For this review, take the finished solid that the model builds, in its own axes (mm). Face numbers are marked on the shaded views. A direction names the side the tool comes from. Give positions to 0.01 mm unless a question says otherwise; leave off trailing zeros. Loops run counter-clockwise (first coordinate to the right, second up) from the corner with the lowest first, then second, coordinate; pieces in that order, holes last.
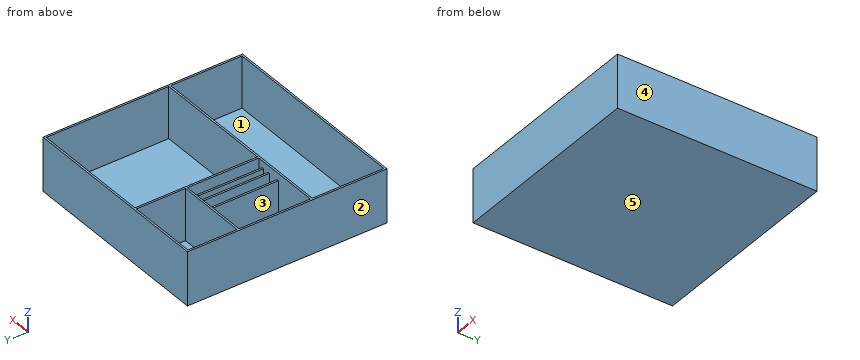
```python
from build123d import *

# Parameters (mm, degrees)
F0_W     = 92
F0_H     = 63.4
F1_DEPTH = 2.4
F0_W_2   = 56.8
F0_H_2   = 92
F0_W_3   = 14
F0_W_4   = 8
F0_W_5   = 6
F0_W_6   = 252.2
F0_W_7   = 257
F0_H_3   = 257
F2_DEPTH = 69
F0_W_8   = 2.4
F3_DEPTH = 60


with BuildPart() as f1:
    # F0 (on Top) → F1 (new body)
    with BuildSketch(Plane.XY):
        with Locations((-80.1, 94.4)):
            Rectangle(F0_W, F0_H)
    extrude(amount=F1_DEPTH)



with BuildPart() as f1b:
    # F0 (on Top) → F1, piece 2 (new body)
    with BuildSketch(Plane.XY):
        with Locations((-97.7, 14.3)):
            Rectangle(F0_W_2, F0_H_2)
    extrude(amount=F1_DEPTH)


with BuildPart() as f1c:
    # F0 (on Top) → F1, piece 3 (new body)
    with BuildSketch(Plane.XY):
        with Locations((-59.9, 14.3)):
            Rectangle(F0_W_3, F0_H_2)
    extrude(amount=F1_DEPTH)


with BuildPart() as f1d:
    # F0 (on Top) → F1, piece 4 (new body)
    with BuildSketch(Plane.XY):
        with Locations((-46.5, 14.3)):
            Rectangle(F0_W_4, F0_H_2)
    extrude(amount=F1_DEPTH)


with BuildPart() as f1e:
    # F0 (on Top) → F1, piece 5 (new body)
    with BuildSketch(Plane.XY):
        with Locations((-37.1, 14.3)):
            Rectangle(F0_W_5, F0_H_2)
    extrude(amount=F1_DEPTH)


with BuildPart() as f1f:
    # F0 (on Top) → F1, piece 6 (new body)
    with BuildSketch(Plane.XY):
        Polygon((126.1, 126.1), (-31.7, 126.1), (-31.7, 60.3), (-31.7, -31.7), (126.1, -31.7), align=None)
    extrude(amount=F1_DEPTH)


with BuildPart() as f1g:
    # F0 (on Top) → F1, piece 7 (new body)
    with BuildSketch(Plane.XY):
        with Locations((0, -80.1)):
            Rectangle(F0_W_6, F0_H_2)
    extrude(amount=F1_DEPTH)


with BuildPart() as f1_1:
    add(f1.part)

    add(f1b.part)  # F2 merges F1b

    add(f1c.part)  # F2 merges F1c

    add(f1d.part)  # F2 merges F1d

    add(f1e.part)  # F2 merges F1e

    add(f1f.part)  # F2 merges F1f

    add(f1g.part)  # F2 merges F1g
    # F0 (on Top) → F2 (join)
    with BuildSketch(Plane.XY):
        Rectangle(F0_W_7, F0_H_3)
        Polygon((-126.1, 62.7), (-126.1, 126.1), (-34.1, 126.1), (-31.7, 126.1), (126.1, 126.1), (126.1, -31.7), (126.1, -34.1), (126.1, -126.1), (-126.1, -126.1), (-126.1, -34.1), (-126.1, -31.7), (-126.1, 60.3), align=None, mode=Mode.SUBTRACT)
        Polygon((-69.3, -31.7), (-126.1, -31.7), (-126.1, -34.1), (126.1, -34.1), (126.1, -31.7), (-31.7, -31.7), (-34.1, -31.7), (-40.1, -31.7), (-42.5, -31.7), (-50.5, -31.7), (-52.9, -31.7), (-66.9, -31.7), align=None)
        Polygon((-34.1, 62.7), (-126.1, 62.7), (-126.1, 60.3), (-69.3, 60.3), (-66.9, 60.3), (-52.9, 60.3), (-50.5, 60.3), (-42.5, 60.3), (-40.1, 60.3), (-34.1, 60.3), align=None)
        Polygon((-31.7, 126.1), (-34.1, 126.1), (-34.1, 62.7), (-34.1, 60.3), (-34.1, -31.7), (-31.7, -31.7), (-31.7, 60.3), align=None)
    extrude(amount=F2_DEPTH)

    # F0 (on Top) → F3 (join)
    with BuildSketch(Plane.XY):
        with Locations((-68.1, 14.3)):
            Rectangle(F0_W_8, F0_H_2)
        with Locations((-51.7, 14.3)):
            Rectangle(F0_W_8, F0_H_2)
        with Locations((-41.3, 14.3)):
            Rectangle(F0_W_8, F0_H_2)
    extrude(amount=F3_DEPTH)


solid = f1_1.part
```
Item 1: Clearance check with flat-ended pins moving along their axes: pin 1 Ø2.5 at (x, y) = (-52, 22.5) entering from +Z; pin 2 Ø1.8 at (x, y) = (-36.5, -3) entering from +Z. State where each tip first meets the part, or that it passes through.
Answer:
pin 1: stops at z = 60
pin 2: stops at z = 2.4
Item 2: Take a section at A-A on z = 11. State how many separate pieces and enclosed holes the cut face has, and give its area (3 significant figures).
Answer:
separate pieces: 1
enclosed holes: 7
area: 4,310 mm2
Item 3: Tool access review of the marked faces 1 and 2: name each direction out of +Z, -Z, +X, -X, +Y, -Y from which nothing blocks a thin tool from reaching the whole face with its end or side.
Answer:
face 1: +Z
face 2: +Z, -Z, -X, +Y, -Y
Item 4: The part is to be moulded in two halves that separate along X. For the marked faces 3, 4 and 5, say which applies: released by +X, released by -X, zero draft, split by the parting line, or undercut.
Answer:
face 3: undercut
face 4: released by +X
face 5: zero draft
Item 5: Take a section at B-B on x = 41. Give the boundary of the cut face in (y, z), and give its area (3 significant figures).
Answer:
outline: (-128.5, 0) - (128.5, 0) - (128.5, 69) - (126.1, 69) - (126.1, 2.4) - (-31.7, 2.4) - (-31.7, 69) - (-34.1, 69) - (-34.1, 2.4) - (-126.1, 2.4) - (-126.1, 69) - (-128.5, 69) - close
area: 1,100 mm2
Item 6: For L1, parallel to Y at x = -12.5, z = 33; L2, parallel to Y at x = -99, z = 39.5; L3, parallel to X at y = -17, z = 13.5, list the stretches that pass through material, from the lowest coordinate up.
Answer:
L1: y = -128.5 to -126.1, -34.1 to -31.7, 126.1 to 128.5
L2: y = -128.5 to -126.1, -34.1 to -31.7, 60.3 to 62.7, 126.1 to 128.5
L3: x = -128.5 to -126.1, -69.3 to -66.9, -52.9 to -50.5, -42.5 to -40.1, -34.1 to -31.7, 126.1 to 128.5
Item 7: Take a section at D-D on y = 32.5. Give the boundary of the cut face in (x, z).
Answer:
outline: (-128.5, 0) - (128.5, 0) - (128.5, 69) - (126.1, 69) - (126.1, 2.4) - (-31.7, 2.4) - (-31.7, 69) - (-34.1, 69) - (-34.1, 2.4) - (-40.1, 2.4) - (-40.1, 60) - (-42.5, 60) - (-42.5, 2.4) - (-50.5, 2.4) - (-50.5, 60) - (-52.9, 60) - (-52.9, 2.4) - (-66.9, 2.4) - (-66.9, 60) - (-69.3, 60) - (-69.3, 2.4) - (-126.1, 2.4) - (-126.1, 69) - (-128.5, 69) - close
Item 8: Take a section at C-C on z = 65.5. Give the boundary of the cut face in (x, y), and give its area (3 significant figures).
Answer:
outline: (-128.5, -128.5) - (128.5, -128.5) - (128.5, 128.5) - (-128.5, 128.5) - close; hole (-126.1, -126.1) - (126.1, -126.1) - (126.1, -34.1) - (-126.1, -34.1) - close; hole (-126.1, -31.7) - (-34.1, -31.7) - (-34.1, 60.3) - (-126.1, 60.3) - close; hole (-126.1, 62.7) - (-34.1, 62.7) - (-34.1, 126.1) - (-126.1, 126.1) - close; hole (-31.7, -31.7) - (126.1, -31.7) - (126.1, 126.1) - (-31.7, 126.1) - close
area: 3,650 mm2
